from build123d import *

# Parameters (mm, degrees)
BOSS_EXTRUDE2_DEPTH = 208
CUT_EXTRUDE1_REACH  = 212.31
SKETCH5_R           = 2.125
SKETCH6_W           = 100
SKETCH6_H           = 100
BOSS_EXTRUDE5_DEPTH = 5
CUT_EXTRUDE2_REACH  = 221.691
SKETCH7_R           = 4.5
SKETCH8_W           = 18
SKETCH8_H           = 23
SKETCH8_W_2         = 12
SKETCH8_H_2         = 15.5
BOSS_EXTRUDE6_DEPTH = 10
CUT_EXTRUDE7_START  = -5
SKETCH10_R          = 4.8
SKETCH10_R_2        = 4.5
CUT_EXTRUDE7_DEPTH  = 5


with BuildPart() as part:
    # Sketch3 → Boss-Extrude2 (new body)
    with BuildSketch(Plane(origin=(0, 0, 0), x_dir=(1, 0, 0), z_dir=(0, 1, 0))):
        Polygon((9, 8.5), (-9, 8.5), (-9, -11.5), (-14, -11.5), (-14, 13.5), (14, 13.5), (14, -11.5), (9, -11.5), align=None)
    extrude(amount=-BOSS_EXTRUDE2_DEPTH)

    # Cut-Extrude1: up to this face of the body (flat: up to its plane)
    cut_extrude1_end = Plane(part.part.faces().sort_by_distance((-14, -104, -1))[0])
    # Sketch5 → Cut-Extrude1 (cut, up to the picked face)
    with BuildSketch(Plane(origin=(14, 0, 0), x_dir=(0, 0, -1), z_dir=(1, 0, 0)), mode=Mode.PRIVATE) as cut_extrude1_sk1:
        with Locations((0, -4.5)):
            Circle(SKETCH5_R)
    cut_extrude1_tool1 = split(extrude(cut_extrude1_sk1.sketch, amount=-CUT_EXTRUDE1_REACH, mode=Mode.PRIVATE), bisect_by=cut_extrude1_end, keep=Keep.BOTH, mode=Mode.PRIVATE)
    add(cut_extrude1_tool1.solids().sort_by(Axis((14, -4.5, 0), (-1, 0, 0)))[0], mode=Mode.SUBTRACT)

    # Sketch6 → Boss-Extrude5 (add)
    with BuildSketch(Plane.XZ.offset(208)):
        Rectangle(SKETCH6_W, SKETCH6_H)
    extrude(amount=BOSS_EXTRUDE5_DEPTH)

    # Sketch7 → Cut-Extrude2 (cut, up to next)
    with BuildSketch(Plane(origin=(0, -208, 0), x_dir=(1, 0, 0), z_dir=(0, 1, 0)), mode=Mode.PRIVATE) as cut_extrude2_sk1:
        with Locations(Location((0, 0, 0), (0, 0, 270))):
            Circle(SKETCH7_R)
    cut_extrude2_tool1 = extrude(cut_extrude2_sk1.sketch, amount=-CUT_EXTRUDE2_REACH, mode=Mode.PRIVATE) & part.part
    add(cut_extrude2_tool1.solids().sort_by_distance((0, -208, 0))[0], mode=Mode.SUBTRACT)

    # Sketch8 → Boss-Extrude6 (add)
    with BuildSketch(Plane(origin=(0, -208, 0), x_dir=(1, 0, 0), z_dir=(0, 1, 0))):
        Rectangle(SKETCH8_W, SKETCH8_H)
        with Locations((0, 1.25)):
            Rectangle(SKETCH8_W_2, SKETCH8_H_2, mode=Mode.SUBTRACT)
    extrude(amount=BOSS_EXTRUDE6_DEPTH)

    # Sketch10 → Cut-Extrude7 (cut)
    with BuildSketch(Plane.XZ.offset(213).offset(CUT_EXTRUDE7_START)):
        with Locations(Location((0, 0, 0), (0, 0, 270))):
            Circle(SKETCH10_R)
        Circle(SKETCH10_R_2, mode=Mode.SUBTRACT)
    extrude(amount=CUT_EXTRUDE7_DEPTH, mode=Mode.SUBTRACT)


solid = part.part
For this review, take the finished solid that the model builds, in its own axes (mm). A direction names the side the tool comes from. Round coordinates to 2 decimals unless told otherwise and drop trailing zeros. Order: outer loops, then holes, each group sorted by start corner. A loop starts at its lowest first (then second) coordinate and runs counter-clockwise, first axis right, second up. Notation, with made-up numbers: M 69.25,-16 L 115.25,-16 A20 cw 115.25,-3 Z; hole C 38,11.5 d1. An arc over 180 degrees is marked long. Use a Markdown table: item, result. Add a question column.
Item 1: Mouldability with a two-part tool opening along Z and no side actions: class faces 1 (the cylindrical face through (4.05, -210.46, -2.58)), 2 (the flat face through (-10, -105, 11.5)), 3 (the flat face through (14, -103, -1)), 4 (the flat face through (0, -103, -13.5)) as released by +Z, released by -Z, zero draft, split by the parting line, or undercut.
Item 2: Add section B-B, the plane x = 0. Give the boundary of the cut face in (y, z), then the cut area to 3 significant figures.
Item 3: Insertion check: pin 1 (7 mm diameter, centred on y = -4.5, z = 0, fed in from -X); pin 2 (8 mm diameter, centred on x = -25, z = 39, fed in from +Y); pin 3 (6 mm diameter, centred on y = -122, z = 1.5, fed in from +X). Each pin has a flat end and moves straight along its axis. Give the tip position at first contact, or say it passes through.
Item 4: Tool access review of faces 5 (the flat face through (-2, -198, 8)), 6 (the flat face through (-6, -203, -1)), 7 (the flat face through (-14, -103, -1)): name each direction out of +Z, -Z, +X, -X, +Y, -Y from which nothing blocks a thin tool from reaching the whole face with its end or side.
Item 5: Add section C-C, the plane y = -4.5. Give the boundary of the cut face in (x, z) (3 decimals), then the cut area to 4 significant figures.
Item 6: Add section A-A, the plane z = 0. Give the boundary of the cut face in (x, y) (3 decimals), then the cut area to 3 significant figures.
Item 7: To check wall thickness, follow line 1 along Y through (x, z) = (10.05, 0) (3 decimals); line 2 along X through (y, z) = (-209, 0); line 3 along X through (y, z) = (-191, 5.5). State the ranges of each line that lie inside material, in increasing order.
Item 8: Add section D-D, the plane y = -179. Give the boundary of the cut face in (x, z), then the cut area to 3 significant figures.
Geometry results:
| question | item | result |
|---|---|---|
| 1 | face 1 | undercut |
| 1 | face 2 | released by +Z |
| 1 | face 3 | zero draft |
| 1 | face 4 | released by -Z |
| 2 | outline | M -213,-50 L -208,-50 L -208,-13.5 L 0,-13.5 L 0,-8.5 L -208,-8.5 L -208,-4.8 L -213,-4.8 Z; M -213,4.8 L -208,4.8 L -208,6.5 L -198,6.5 L -198,11.5 L -208,11.5 L -208,50 L -213,50 Z |
| 2 | area | 1,540 mm² |
| 3 | pin 1 | stops at x = -14 |
| 3 | pin 2 | stops at y = -208 |
| 3 | pin 3 | stops at x = 14 |
| 4 | face 5 | +Z, +Y |
| 4 | face 6 | +Y |
| 4 | face 7 | +Z, -Z, -X, +Y |
| 5 | outline | M -14,-13.5 L 14,-13.5 L 14,-2.125 L 9,-2.125 L 9,-8.5 L -9,-8.5 L -9,-2.125 L -14,-2.125 Z; M -14,2.125 L -9,2.125 L -9,11.5 L -14,11.5 Z; M 9,2.125 L 14,2.125 L 14,11.5 L 9,11.5 Z |
| 5 | area | 297.5 mm² |
| 6 | outline | M -50,-213 L -4.8,-213 L -4.8,-208 L -6,-208 L -6,-198 L -9,-198 L -9,-6.625 L -14,-6.625 L -14,-208 L -50,-208 Z; M -14,-2.375 L -9,-2.375 L -9,0 L -14,0 Z; M 4.8,-213 L 50,-213 L 50,-208 L 14,-208 L 14,-6.625 L 9,-6.625 L 9,-198 L 6,-198 L 6,-208 L 4.8,-208 Z; M 9,-2.375 L 14,-2.375 L 14,0 L 9,0 Z |
| 6 | area | 2,550 mm² |
| 7 | line 1 | y = -213 to -6.625, -2.375 to 0 |
| 7 | line 2 | x = -50 to -4.8, 4.8 to 50 |
| 7 | line 3 | x = -14 to -9, 9 to 14 |
| 8 | outline | M -14,-13.5 L 14,-13.5 L 14,11.5 L 9,11.5 L 9,-8.5 L -9,-8.5 L -9,11.5 L -14,11.5 Z |
| 8 | area | 340 mm² |
